```python
from build123d import *

# Parameters (mm, degrees)
F1_DEPTH = 584.2
F3_W     = 25.4
F3_H     = 3.175
F3_W_2   = 6.35
F3_H_2   = 9.525
F4_DEPTH = 68.58
F6_D     = 9.525


with BuildPart() as f1:
    # F0 (on Front) → F1 (new body, symmetric)
    with BuildSketch(Plane.XZ):
        Polygon((17.960512, 0), (21.328108, 0), (0, 21.328108), (-21.328108, 0), (-17.960512, 0), (0, 17.960512), align=None)
    extrude(amount=F1_DEPTH, both=True)

    # F3 (on offset) → F4 (cut)
    with BuildSketch(Plane.YZ.offset(37.592)):
        with Locations((-558.8, 19.740608)):
            Rectangle(F3_W, F3_H)
        with Locations((558.8, 19.740608)):
            Rectangle(F3_W, F3_H)
        with Locations((581.025, 4.7625)):
            Rectangle(F3_W_2, F3_H_2)
        with Locations((-581.025, 4.7625)):
            Rectangle(F3_W_2, F3_H_2)
    extrude(amount=-F4_DEPTH, mode=Mode.SUBTRACT)

    # F6 (through all)
    with Locations(Plane.XY.offset(18.153108)):
        with Locations((0, -558.8), (0, 558.8)):
            Hole(F6_D / 2)


solid = f1.part
```
Read the model definition and answer for the solid it produces. Units are mm, in the model's axes. Round coordinates to 2 decimals unless told otherwise and drop trailing zeros. Write each loop counter-clockwise with the first axis right and the second up, starting at its lowest first coordinate (ties: lowest second). Pieces come first, ordered by that corner, then holes. Notation, with made-up numbers: (-1, 70) -> (9, 70) arc R13 ccw to (9, 77) -> close; hole circle Ø7 at (-36.75, -15). An arc over 180 degrees is marked (long way). Answer in a Markdown table with one row per item. Add a question column.
1) Determine the mould class of faces 1 (the face through (10.813, -8.179, 10.515)), 2 (the face through (8.85, -8.18, 9.11)), 3 (the face through (-10.515, -8.179, 10.813)) for opening direction X: pulls with the +X half, pulls with the -X half, needs draft (parallel to the pull), parting line crosses it, or undercut.
2) Find section B-B, the plane y = 479. Determine the outline of the cut face in (x, z).
3) Given P1, Ø2, axis at y = 299, z = 11, coming from the +X side; P2, Ø1.9, axis at x = 0.5, y = 565, coming from the +Z side; P3, Ø5, axis at x = -17, z = 4.5, coming from the +Y side, each flat-ended and moving along its own axis, determine where each tip first touches the part or whether it passes through.
4) Consider line 1 (Y direction, x = 1.5, z = 19); line 2 (X direction, y = -463.5, z = 9.5); line 3 (X direction, y = 281.5, z = 6.25). Determine where each line is inside the solid, lowest interval first.
5) Find section A-A, the plane z = 5.5. Determine the outline of the cut face in (x, y).
Findings below:
| question | item | result |
|---|---|---|
| 1 | face 1 | pulls with the +X half |
| 1 | face 2 | undercut |
| 1 | face 3 | pulls with the -X half |
| 2 | outline | (-21.33, 0) -> (-17.96, 0) -> (0, 17.96) -> (17.96, 0) -> (21.33, 0) -> (0, 21.33) -> close |
| 3 | P1 | x = 11.33 |
| 3 | P2 | z = 18.15 |
| 3 | P3 | y = 577.85 |
| 4 | line 1 | -584.2 to -571.5, -546.1 to 546.1, 571.5 to 584.2 |
| 4 | line 2 | -11.83 to -8.46, 8.46 to 11.83 |
| 4 | line 3 | -15.08 to -11.71, 11.71 to 15.08 |
| 5 | outline | (-15.83, -577.85) -> (-12.46, -577.85) -> (-12.46, 577.85) -> (-15.83, 577.85) -> close; (12.46, -577.85) -> (15.83, -577.85) -> (15.83, 577.85) -> (12.46, 577.85) -> close |
